Model file for the job. Use its own axes, mm. A direction names the side the tool comes from. Give positions to 0.01 mm unless a question says otherwise; leave off trailing zeros. Write each loop counter-clockwise with the first axis right and the second up, starting at its lowest first coordinate (ties: lowest second). Pieces come first, ordered by that corner, then holes. Notation, with made-up numbers: (50.25, 1.25) - (77.25, 1.25) arc R7 ccw to (77.25, 14.25) - close; hole circle Ø8 at (58, -4.5). An arc over 180 degrees is marked (long way). Use CSV: the item, a comma, the result in double quotes.
from build123d import *

# Parameters (mm, degrees)
CROQUIS1_R              = 12
CROQUIS1_R_2            = 1.25
SALIENTE_EXTRUIR1_DEPTH = 3
SALIENTE_EXTRUIR2_START = 3
CROQUIS1_3_R            = 3
SALIENTE_EXTRUIR2_DEPTH = 10
CORTAR_EXTRUIR1_START   = -5
CORTAR_EXTRUIR1_DEPTH   = 5
CHAFL_N1_SIZE           = 0.5


with BuildPart() as part:
    # Croquis1 → Saliente-Extruir1 (new body)
    with BuildSketch(Plane(origin=(0, 0, 0), x_dir=(1, 0, 0), z_dir=(0, 1, 0))):
        with Locations(Location((0, 0, 0), (0, 0, 270))):
            Circle(CROQUIS1_R)
        with Locations(Location((-6.576093065, 6.576093065, 0), (0, 0, 270))):
            Circle(CROQUIS1_R_2, mode=Mode.SUBTRACT)
        with Locations(Location((5.656854249, 5.656854249, 0), (0, 0, 270))):
            Circle(CROQUIS1_R_2, mode=Mode.SUBTRACT)
        with Locations(Location((6.576093065, -6.576093065, 0), (0, 0, 270))):
            Circle(CROQUIS1_R_2, mode=Mode.SUBTRACT)
        with Locations(Location((-5.656854249, -5.656854249, 0), (0, 0, 270))):
            Circle(CROQUIS1_R_2, mode=Mode.SUBTRACT)
    extrude(amount=SALIENTE_EXTRUIR1_DEPTH)

    # Croquis1<3> → Saliente-Extruir2 (add)
    with BuildSketch(Plane(origin=(0, 0, 0), x_dir=(1, 0, 0), z_dir=(0, 1, 0)).offset(SALIENTE_EXTRUIR2_START)):
        with Locations(Location((0, 0, 0), (0, 0, 270))):
            Circle(CROQUIS1_3_R)
    extrude(amount=SALIENTE_EXTRUIR2_DEPTH)

    # Croquis2 → Cortar-Extruir1 (cut)
    with BuildSketch(Plane(origin=(0, 13, 0), x_dir=(1, 0, 0), z_dir=(0, 1, 0)).offset(CORTAR_EXTRUIR1_START)):
        with BuildLine():
            Line((1.5, 2.598076211), (1.5, -2.598076211))
            ThreePointArc((1.5, -2.598076211), (3, 0), (1.5, 2.598076211))
        make_face()
    extrude(amount=CORTAR_EXTRUIR1_DEPTH, mode=Mode.SUBTRACT)

    # Chaflán1
    chafl_n1_edges = [part.edges().sort_by_distance(p)[0] for p in [
        (-2.897777479, 13, -0.776457135),
    ]]
    chamfer(chafl_n1_edges, length=CHAFL_N1_SIZE)


solid = part.part
(1) Saw through at A-A, the plane z = 0. List the corners of the cut face in (x, y), then the cut area to 3 significant figures.
Checked values:
outline,"(-12, 0) - (12, 0) - (12, 3) - (3, 3) - (3, 8) - (1.5, 8) - (1.5, 13) - (-2.5, 13) - (-3, 12.5) - (-3, 3) - (-12, 3) - close"
area,"124 mm^2"
(2) Saw through at B-B, the plane x = 0. List the corners of the cut face in (y, z).
Checked values:
outline,"(0, -12) - (3, -12) - (3, -3) - (12.5, -3) - (13, -2.5) - (13, 2.5) - (12.5, 3) - (3, 3) - (3, 12) - (0, 12) - close"
(3) Flat gauge pins, fed straight in: P1, Ø2, axis at y = 6.5, z = 2.5, coming from the -X side; P2, Ø1.2, axis at x = 2.5, z = -0.5, coming from the +Y side; P3, Ø2, axis at x = 5.66, z = -5.66, coming from the +Y side; P4, Ø3, axis at x = -6.58, z = -6.58, coming from the +Y side. Where does each tip first touch, or does it go through?
Checked values:
P1,"stops at x = -2.6"
P2,"stops at y = 8"
P3,"passes through"
P4,"stops at y = 3"
(4) Wall check: probe 1 along Y at (x, z) = (6.25, -9); probe 2 along Z at (x, y) = (5.25, 2.5); probe 3 along Z at (x, y) = (8.75, 2.5). Give the ranges that are in metal, low to high. Write a range as [from, to].
Checked values:
probe 1,"y = [0, 3]"
probe 2,"z = [-10.79, -6.84], [-4.47, 10.79]"
probe 3,"z = [-8.21, 8.21]"
(5) Saw through at D-D, the plane y = 6. List the corners of the cut face in (x, z), then the cut area to 3 significant figures.
Checked values:
outline,"circle Ø6 at (0, 0)"
area,"28.3 mm^2"
(6) Saw through at C-C, the plane y = 1.5. List the corners of the cut face in (x, z).
Checked values:
outline,"circle Ø24 at (0, 0); hole circle Ø2.5 at (-6.58, -6.58); hole circle Ø2.5 at (-5.66, 5.66); hole circle Ø2.5 at (5.66, -5.66); hole circle Ø2.5 at (6.58, 6.58)"
(7) 3-axis set-ups, long thin cutter, end or side, ignore diameter. For faces 4 (the face through (0, 13, 0)), 5 (the face through (-2.5, 3, 2.5)), 6 (the face through (2, 8, 0)): which of +Z, -Z, +X, -X, +Y, -Y reach the whole face in a straight line?
Checked values:
face 4,"+Z, -Z, +X, -X, +Y"
face 5,"+Y"
face 6,"+Z, -Z, +X, +Y"
(8) Pull direction X, two halves, no side cores. Call faces 1 (the face through (1.5, 10, 0)), 2 (the face through (-2.93, 7.68, -0.65)), 3 (the face through (6.631, 1.479, 5.327)): released by +X, released by -X, zero draft, split by the parting line, or undercut.
Checked values:
face 1,"released by +X"
face 2,"split by the parting line"
face 3,"undercut"
